Geometry check sheet. Reference: drawing and pictorial views, mm from the part's lowest x, y, z. A direction names the side the tool comes from. Give positions to 0.01 mm unless a question says otherwise; leave off trailing zeros. Order: outer loops, then holes, each group sorted by start corner. A loop starts at its lowest first (then second) coordinate and runs counter-clockwise, first axis right, second up.
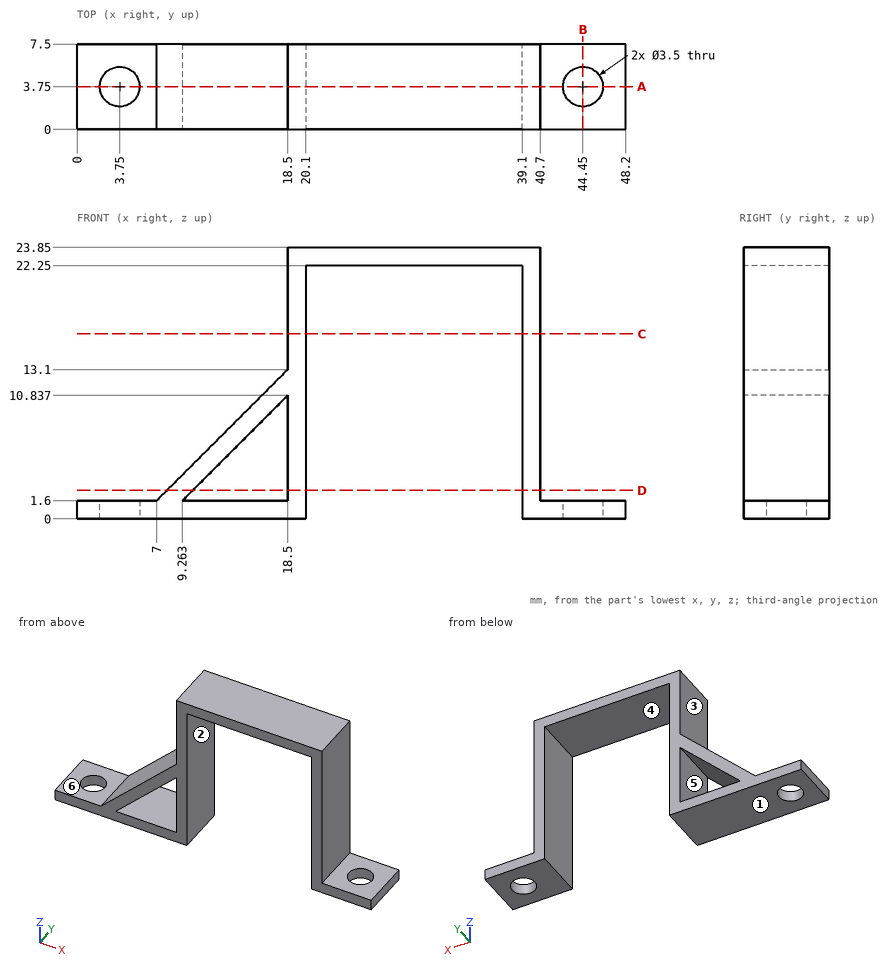
1) Section check D-D, the plane z = 2.5. Record the cut outline in (x, y).
Recorded:
outline: (7.9, 0) - (10.16, 0) - (10.16, 7.5) - (7.9, 7.5) - close; (18.5, 0) - (20.1, 0) - (20.1, 7.5) - (18.5, 7.5) - close; (39.1, 0) - (40.7, 0) - (40.7, 7.5) - (39.1, 7.5) - close
2) Draft check along X on the marked faces 1, 2 and 3. Enter one of: +X half, -X half, draft (parallel to the pull), parting line (faces both ways), or undercut.
Recorded:
face 1: draft
face 2: undercut
face 3: -X half
3) Depth check by flat-ended pin: pin 1 Ø4 at (y, z) = (2.5, 9) entering from +X; pin 2 Ø4 at (x, y) = (44.45, 3.75) entering from +Z; pin 3 Ø2 at (x, z) = (36.5, 12) entering from -Y; pin 4 Ø4 at (x, y) = (33.5, 4.5) entering from -Z. Enter the tip coordinate at first touch or a pass-through.
Recorded:
pin 1: stops at x = 40.7
pin 2: stops at z = 1.6
pin 3: passes through
pin 4: stops at z = 22.25
4) Set-up check for the marked faces 4, 5 and 6: record each of +Z, -Z, +X, -X, +Y, -Y from which the full face is reachable in a straight line by a thin tool's end or side.
Recorded:
face 4: -Z, +Y, -Y
face 5: +Y, -Y
face 6: +Z, -X, +Y, -Y
5) Section check B-B, the plane x = 44.45. Record the cut outline in (y, z).
Recorded:
outline: (0, 0) - (2, 0) - (2, 1.6) - (0, 1.6) - close; (5.5, 0) - (7.5, 0) - (7.5, 1.6) - (5.5, 1.6) - close
6) Section check C-C, the plane z = 16.25. Record the cut outline in (x, y).
Recorded:
outline: (18.5, 0) - (20.1, 0) - (20.1, 7.5) - (18.5, 7.5) - close; (39.1, 0) - (40.7, 0) - (40.7, 7.5) - (39.1, 7.5) - close
7) Material ranges on L1, parallel to Y at x = 3.75, z = 0.65; L2, parallel to X at y = 3.5, z = 15.5; L3, parallel to X at y = 5, z = 4.75, recorded low to high.
Recorded:
L1: y = 0 to 2, 5.5 to 7.5
L2: x = 18.5 to 20.1, 39.1 to 40.7
L3: x = 10.15 to 12.41, 18.5 to 20.1, 39.1 to 40.7
8) Section check A-A, the plane y = 3.75. Record the cut outline in (x, z).
Recorded:
outline: (0, 0) - (2, 0) - (2, 1.6) - (0, 1.6) - close; (5.5, 0) - (20.1, 0) - (20.1, 22.25) - (39.1, 22.25) - (39.1, 0) - (42.7, 0) - (42.7, 1.6) - (40.7, 1.6) - (40.7, 23.85) - (18.5, 23.85) - (18.5, 13.1) - (7, 1.6) - (5.5, 1.6) - close; (46.2, 0) - (48.2, 0) - (48.2, 1.6) - (46.2, 1.6) - close; hole (9.26, 1.6) - (18.5, 1.6) - (18.5, 10.84) - close
